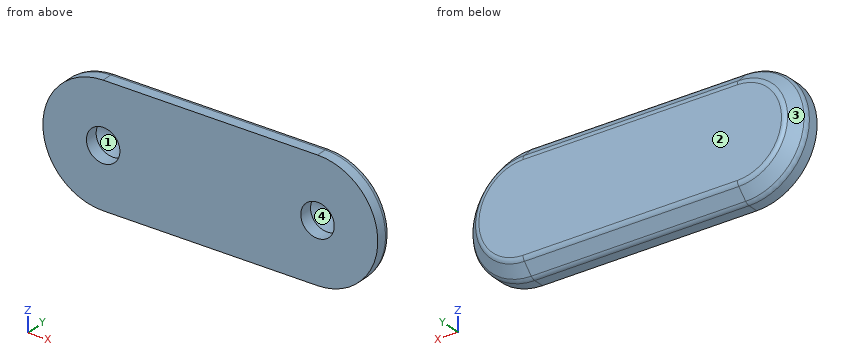
from build123d import *

# Parameters (mm, degrees)
BOSS_EXTRUDE1_DEPTH             = 2
TAP_DRILL_FOR_M3X0_5_TAP1_D     = 2.5
TAP_DRILL_FOR_M3X0_5_TAP1_DEPTH = 1
TAP_DRILL_FOR_M3X0_5_TAP1_TIP   = 0.751075774
CHAMFER3_SIZE                   = 1
FILLET1_R                       = 0.5


with BuildPart() as part:
    # Sketch1 → Boss-Extrude1 (new body)
    with BuildSketch(Plane(origin=(0, 0, 0), x_dir=(1, 0, 0), z_dir=(0, 1, 0))):
        with BuildLine():
            Line((8, -4.5), (-8, -4.5))
            ThreePointArc((-8, -4.5), (-12.5, 0), (-8, 4.5))
            Line((-8, 4.5), (8, 4.5))
            ThreePointArc((8, 4.5), (12.5, 0), (8, -4.5))
        make_face()
    extrude(amount=BOSS_EXTRUDE1_DEPTH)

    # Tap Drill for M3x0.5 Tap1
    with Locations(Plane.XZ):
        with Locations((-8, 0), (8, 0)):
            Hole(TAP_DRILL_FOR_M3X0_5_TAP1_D / 2, depth=TAP_DRILL_FOR_M3X0_5_TAP1_DEPTH)
            with Locations((0, 0, -(TAP_DRILL_FOR_M3X0_5_TAP1_DEPTH + TAP_DRILL_FOR_M3X0_5_TAP1_TIP / 2))):  # 118° drill point
                Cone(0, TAP_DRILL_FOR_M3X0_5_TAP1_D / 2, TAP_DRILL_FOR_M3X0_5_TAP1_TIP, mode=Mode.SUBTRACT)

    # Chamfer3
    chamfer3_edges = [part.edges().sort_by_distance(p)[0] for p in [
        (12.5, 2, 0),
        (0, 2, -4.5),
        (-12.5, 2, 0),
        (0, 2, 4.5),
    ]]
    chamfer(chamfer3_edges, length=CHAMFER3_SIZE)

    # Fillet1
    fillet1_edges = [part.edges().sort_by_distance(p)[0] for p in [
        (0, 2, 3.5),
        (11.5, 2, 0),
        (-11.5, 2, 0),
        (0, 2, -3.5),
        (0, 1, -4.5),
        (-12.5, 1, 0),
        (12.5, 1, 0),
        (0, 1, 4.5),
    ]]
    fillet(fillet1_edges, radius=FILLET1_R)


solid = part.part
Work out the finished part from the listing and answer in its coordinate system (mm). Face numbers are marked on the shaded views. Give positions to 0.01 mm unless a question says otherwise; leave off trailing zeros. Write each loop counter-clockwise with the first axis right and the second up, starting at its lowest first coordinate (ties: lowest second). Pieces come first, ordered by that corner, then holes.
Q1. Given pin 1 (2 mm diameter, centred on x = -8, z = 0, fed in from -Y), flat-ended and moving along its own axis, determine where the tip first touches the part or whether it passes through.
Answer:
pin 1: stops at y = 1.15
Q2. Straight lines are drawn through the part: L1, parallel to X at y = 0.6, z = 0; L2, parallel to Z at x = 8, y = 0.75; L3, parallel to X at y = 1.3, z = 0.5. For each, find the intervals that lie inside material, in ascending order.
Answer:
L1: x = -12.5 to -9.25, -6.75 to 6.75, 9.25 to 12.5
L2: z = -4.5 to -1.25, 1.25 to 4.5
L3: x = -12.17 to -8.56, -7.44 to 7.44, 8.56 to 12.17
Q3. For a pull along Z with two mould halves and no side action, classify the marked faces 1, 2, 3 and 4 as released by +Z, released by -Z, zero draft, split by the parting line, or undercut.
Answer:
face 1: undercut
face 2: zero draft
face 3: split by the parting line
face 4: undercut
Q4. The part is cut by section B-B on y = 1.5. Give the vertices of the cut face in (x, z).
Answer:
outline: (-8, -4) - (8, -4) arc R4 ccw to (8, 4) - (-8, 4) arc R4 ccw to start; hole circle Ø0.84 at (-8, 0); hole circle Ø0.84 at (8, 0)
Q5. The part is cut by section A-A on x = 1.5. Give the vertices of the cut face in (y, z).
Answer:
outline: (0, -4.5) - (0.79, -4.5) arc R0.5 ccw to (1.15, -4.35) - (1.85, -3.65) arc R0.5 ccw to (2, -3.29) - (2, 3.29) arc R0.5 ccw to (1.85, 3.65) - (1.15, 4.35) arc R0.5 ccw to (0.79, 4.5) - (0, 4.5) - close
